Source: CAD feature listing. Evaluate the final solid. Frame: model axes, mm. A direction names the side the tool comes from. Give positions to 0.01 mm unless a question says otherwise; leave off trailing zeros. Order: outer loops, then holes, each group sorted by start corner. A loop starts at its lowest first (then second) coordinate and runs counter-clockwise, first axis right, second up. Notation, with made-up numbers: M 23,-21.75 L 49,-21.75 A27 cw 49,9.25 Z; hole C 66,49.5 d8. An arc over 180 degrees is marked long. Return JSON: item names as keys, results as strings.
from build123d import *

# Parameters (mm, degrees)
F2_R     = 11
F2_R_2   = 5.4
F2_R_3   = 3.9
F3_DEPTH = 1
F4_DEPTH = 3
F5_DEPTH = 0.25
F6_R     = 0.5


# Not quite as in the source:
# - a feature names something its author has since deleted; it is built from what else it names


with BuildPart() as f3:
    # F2 (on Top) → F3 (new body)
    with BuildSketch(Plane.XY):
        Circle(F2_R)
        Circle(F2_R_2, mode=Mode.SUBTRACT)
        Circle(F2_R_2)
        Circle(F2_R_3, mode=Mode.SUBTRACT)
        Circle(F2_R_3)
    extrude(amount=-F3_DEPTH)

    # F2 (on Top) → F4 (join)
    with BuildSketch(Plane.XY):
        Circle(F2_R_3)
    extrude(amount=F4_DEPTH)

    # F2 (on Top) → F5 (join)
    with BuildSketch(Plane.XY):
        Circle(F2_R_2)
        Circle(F2_R_3, mode=Mode.SUBTRACT)
    extrude(amount=F5_DEPTH)

    # F6
    f6_edges = [f3.edges().sort_by_distance(p)[0] for p in [
        (-3.9, 0, 3),
    ]]
    fillet(f6_edges, radius=F6_R)


solid = f3.part
1. Section query A-A (y = 0). Return loops of the section in (x, z), then the cut area to 3 significant figures.
Evaluation:
{"outline": "M -11,-1 L 11,-1 L 11,0 L 5.4,0 L 5.4,0.25 L 3.9,0.25 L 3.9,2.5 A0.5 ccw 3.4,3 L -3.4,3 A0.5 ccw -3.9,2.5 L -3.9,0.25 L -5.4,0.25 L -5.4,0 L -11,0 Z", "area": "46.0 mm^2"}
2. Section query C-C (z = -0.35). Return loops of the section in (x, y).
Evaluation:
{"outline": "C 0,0 d22"}
3. Ray query, probe 1 along Z at (x, y) = (4.75, 4.25); probe 2 along Y at (x, z) = (-0.25, 0.2); probe 3 along Z at (x, y) = (3.75, 2). Return the intervals inside material, ascending.
Evaluation:
{"probe 1": "z = -1 to 0", "probe 2": "y = -5.39 to 5.39", "probe 3": "z = -1 to 0.25"}
4. Section query D-D (z = 1.45). Return loops of the section in (x, y).
Evaluation:
{"outline": "C 0,0 d7.8"}
5. Draft query along Y for faces 3 (the face through (-2.87, 2.64, 1.36)), 4 (the face through (2, -4, 0.25)). Return one class per face: pulls with the +Y half, pulls with the -Y half, needs draft (parallel to the pull), parting line crosses it, or undercut.
Evaluation:
{"face 3": "parting line crosses it", "face 4": "needs draft"}
6. Set-up query: faces 1 (the face through (-3, -5, 0)), 2 (the face through (0, 0, -1)). Return all of +Z, -Z, +X, -X, +Y, -Y with unobstructed straight access to the full face (end or side cutting, diameter ignored); none if empty.
Evaluation:
{"face 1": "+Z", "face 2": "-Z, +X, -X, +Y, -Y"}
